Autodesk Inventor part; units mm, degrees
ref_plane "YZ Plane" through (0, 0, 0) normal (1, 0, 0) x (0, 1, 0)
ref_plane "XZ Plane" through (0, 0, 0) normal (0, 1, 0) x (-1, 0, 0)
ref_plane "XY Plane" through (0, 0, 0) normal (0, 0, 1) x (1, 0, 0)
sketch "Sketch1" plane through (0, 0, 0) normal (0, 0, 1) x (1, 0, 0)
  line L0 (0, 0) -> (76.2, 0)
  line L1 (76.2, 0) -> (76.2, 127)
  line L2 (76.2, 127) -> (0, 127)
  line L3 (0, 127) -> (0, 0)
  dimension "d0" = 76.2
  dimension "d1" = 127
extrude "Extrusion1" add sketch "Sketch1" along normal blind 1244.6
shell "Shell1" thickness 3.175 removed faces 2 at (50.8, 42.3333, 0) at (50.8, 42.3333, 1244.6)
fillet "Fillet1" radius 3.175 8 edges at (0, 127, 622.3) (3.175, 3.175, 622.3) (73.025, 3.175, 622.3) (3.175, 123.825, 622.3) (73.025, 123.825, 622.3) (76.2, 127, 622.3) (0, 0, 622.3) (76.2, 0, 622.3)
sketch "Sketch2" plane through (6.35, 3.175, 0) normal (0, 1, 0) x (1, 0, 0)
  line L0 (-6.35, 0) -> (69.85, 0)
  line L1 (69.85, 0) -> (69.85, -76.2)
  line L2 (69.85, -76.2) -> (-6.35, -76.2)
  line L3 (-6.35, -76.2) -> (-6.35, 0)
  line L4 (51.75, -11.6) -> (11.75, -11.6) construction
  line L5 (11.75, -11.6) -> (11.75, -64.6) construction
  line L6 (11.75, -64.6) -> (51.75, -64.6)
  line L7 (51.75, -64.6) -> (51.75, -11.6) construction
  circle A0 centre (11.75, -64.6) radius 4
  circle A1 centre (11.75, -11.6) radius 4
  circle A2 centre (51.75, -64.6) radius 4
  circle A3 centre (51.75, -11.6) radius 4
  circle A4 centre (31.75, -38.1) radius 4
  circle A5 centre (31.75, -1206.5) radius 4
  line L8 (51.75, -1180) -> (11.75, -1180) construction
  line L9 (11.75, -1180) -> (11.75, -1233) construction
  line L10 (-6.35, -1168.4) -> (69.85, -1168.4)
  line L11 (-6.35, -1244.6) -> (-6.35, -1168.4)
  circle A6 centre (11.75, -1180) radius 4
  line L12 (51.75, -1233) -> (51.75, -1180) construction
  line L13 (69.85, -1168.4) -> (69.85, -1244.6)
  circle A7 centre (51.75, -1180) radius 4
  line L14 (11.75, -1233) -> (51.75, -1233)
  circle A8 centre (11.75, -1233) radius 4
  line L15 (69.85, -1244.6) -> (-6.35, -1244.6)
  circle A9 centre (51.75, -1233) radius 4
  point P0 (31.75, -64.6)
  point P1 (31.75, -76.2)
  point P2 (51.75, -38.1)
  point P3 (69.85, -38.1)
  point P4 (51.75, -1206.5)
  point P5 (69.85, -1206.5)
  point P6 (31.75, -1233)
  point P7 (31.75, -1244.6)
  dimension "d6" = 76.2
  dimension "d7" = 76.2
  dimension "d8" = 53
  dimension "d9" = 40
  dimension "d10" = 8
  dimension "d13" = 1168.4
extrude "Extrusion2" cut sketch "Sketch2" against normal up to surface (3.175 mm away) contours A2 | A0 | A1 | A3 | A4 | A5 | A6 | A7 | A9 | A8
properties part number "2x3_Tube"
Work out the finished part from the listing and answer in its coordinate system (mm). A direction names the side the tool comes from. Round coordinates to 2 decimals unless told otherwise and drop trailing zeros. Order: outer loops, then holes, each group sorted by start corner. A loop starts at its lowest first (then second) coordinate and runs counter-clockwise, first axis right, second up.
Q1. Find the intervals of material crossed by line 1 along Z through (x, y) = (18.1, 1.4); line 2 along X through (y, z) = (2, 1233); line 3 along Z through (x, y) = (38, 1), in increasing order.
Solution:
line 1: z = 0 to 7.6, 15.6 to 60.6, 68.6 to 1176, 1184 to 1229, 1237 to 1244.6
line 2: x = 0.23 to 14.1, 22.1 to 54.1, 62.1 to 75.97
line 3: z = 0 to 34.1, 42.1 to 1202.5, 1210.5 to 1244.6
Q2. The mould has two halves that part along Y. Classify faces 3 (the flat face through (39, 127, 614)), 4 (the flat face through (0, 64, 614)), 5 (the flat face through (73.025, 63, 614)), 6 (the flat face through (38, 0, 614)): pulls with the +Y half, pulls with the -Y half, needs draft (parallel to the pull), parting line crosses it, or undercut.
Solution:
face 3: pulls with the +Y half
face 4: needs draft
face 5: undercut
face 6: pulls with the -Y half
Q3. Given pin 1 Ø1 at (x, z) = (22.5, 937) entering from -Y; pin 2 Ø12 at (x, y) = (14.5, 26.5) entering from -Z; pin 3 Ø5 at (x, z) = (38.1, 1206.5) entering from -Y (3 decimals), each flat-ended and moving along its own axis, determine where each tip first touches the part or whether it passes through.
Solution:
pin 1: stops at y = 0
pin 2: passes through
pin 3: stops at y = 123.825
Q4. A cutting plane is placed at B-B, the plane z = 705. Determine the outline of the cut face in (x, y) (3 decimals).
Solution:
outline: (0, 3.175) arc R3.175 ccw to (3.175, 0) - (73.025, 0) arc R3.175 ccw to (76.2, 3.175) - (76.2, 123.825) arc R3.175 ccw to (73.025, 127) - (3.175, 127) arc R3.175 ccw to (0, 123.825) - close; hole (3.175, 6.35) arc R3.175 ccw to (6.35, 3.175) - (69.85, 3.175) arc R3.175 ccw to (73.025, 6.35) - (73.025, 120.65) arc R3.175 ccw to (69.85, 123.825) - (6.35, 123.825) arc R3.175 ccw to (3.175, 120.65) - close
Q5. A tool of negligible diameter and unlimited length cuts with its end or side. For faces 1 (the flat face through (39, 123.825, 614)), 2 (the flat face through (1, 64, 1244.6)), from which of +Z, -Z, +X, -X, +Y, -Y can it reach the whole face along a straight path? Write none if from no direction.
Solution:
face 1: +Z, -Z
face 2: +Z, +X, -X, +Y, -Y
Q6. A cutting plane is placed at A-A, the plane y = 91. Determine the outline of the cut face in (x, z) (3 decimals).
Solution:
outline: (0, 0) - (3.175, 0) - (3.175, 1244.6) - (0, 1244.6) - close; (73.025, 0) - (76.2, 0) - (76.2, 1244.6) - (73.025, 1244.6) - close
